```python
from build123d import *

# Parameters (mm, degrees)
F2_R         = 10
F2_R_2       = 7.5
F2_R_3       = 4.9
F3_DEPTH     = 11
F4_DEPTH     = 9
F5_DEPTH     = 18.5
F2_R_4       = 11.25
F10_DEPTH    = 1
F11_START    = 9
F10_FACE_R   = 11.25
F10_FACE_R_2 = 10
F11_DEPTH    = 1
F12_DEPTH    = 12


with BuildPart() as f3:
    # F2 (on Top) → F3 (new body)
    with BuildSketch(Plane.XY):
        Circle(F2_R)
        Circle(F2_R_2, mode=Mode.SUBTRACT)
        Circle(F2_R_2)
        Circle(F2_R_3, mode=Mode.SUBTRACT)
        Circle(F2_R_3)
        with BuildLine():
            ThreePointArc((-2.2847319318, -2.45), (-3.35, 0), (-2.2847319318, 2.45))
            Line((-2.2847319318, 2.45), (2.2847319318, 2.45))
            ThreePointArc((2.2847319318, 2.45), (3.35, 0), (2.2847319318, -2.45))
            Line((2.2847319318, -2.45), (-2.2847319318, -2.45))
        make_face(mode=Mode.SUBTRACT)
    extrude(amount=F3_DEPTH)

    # F2 (on Top) → F4 (join)
    with BuildSketch(Plane.XY):
        Circle(F2_R_2)
        Circle(F2_R_3, mode=Mode.SUBTRACT)
        Circle(F2_R_3)
        with BuildLine():
            ThreePointArc((-2.2847319318, -2.45), (-3.35, 0), (-2.2847319318, 2.45))
            Line((-2.2847319318, 2.45), (2.2847319318, 2.45))
            ThreePointArc((2.2847319318, 2.45), (3.35, 0), (2.2847319318, -2.45))
            Line((2.2847319318, -2.45), (-2.2847319318, -2.45))
        make_face(mode=Mode.SUBTRACT)
    extrude(amount=F4_DEPTH)

    # F2 (on Top) → F5 (join)
    with BuildSketch(Plane.XY):
        Circle(F2_R_3)
        with BuildLine():
            ThreePointArc((-2.2847319318, -2.45), (-3.35, 0), (-2.2847319318, 2.45))
            Line((-2.2847319318, 2.45), (2.2847319318, 2.45))
            ThreePointArc((2.2847319318, 2.45), (3.35, 0), (2.2847319318, -2.45))
            Line((2.2847319318, -2.45), (-2.2847319318, -2.45))
        make_face(mode=Mode.SUBTRACT)
    extrude(amount=F5_DEPTH)

    # F6 (on Front) → F7 (revolve)
    with BuildSketch(Plane.XZ):
        Polygon((5.15, 17.75), (4.9, 18.5), (4.9, 17), align=None)
    revolve(axis=Axis((0, 0, 8.7542282417), (0, 0, 1)))

    # F2 (on Top) → F10 (join)
    with BuildSketch(Plane.XY):
        Circle(F2_R_4)
        Circle(F2_R, mode=Mode.SUBTRACT)
    extrude(amount=F10_DEPTH)

    # F2 (on Top) + F10_face (on face) → F11 (join)
    with BuildSketch(Plane.XY.offset(F11_START)):
        Circle(F2_R)
        Circle(F2_R_2, mode=Mode.SUBTRACT)
    with BuildSketch(Plane.XY.offset(1).offset(F11_START)):
        Circle(F10_FACE_R)
        Circle(F10_FACE_R_2, mode=Mode.SUBTRACT)
    extrude(amount=F11_DEPTH)

    # F2 (on Top) → F12 (join)
    with BuildSketch(Plane.XY):
        Circle(F2_R_2)
        Circle(F2_R_3, mode=Mode.SUBTRACT)
    extrude(amount=F12_DEPTH)


solid = f3.part
```
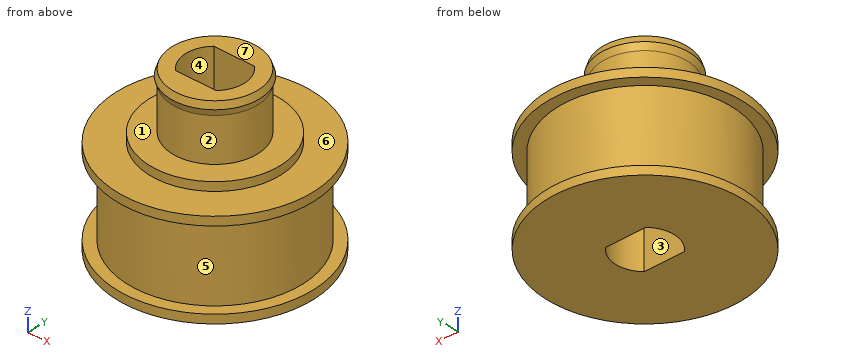
The listing builds one solid part. Answer for the finished solid, in the listing's coordinates (mm). Face numbers are marked on the shaded views. A direction names the side the tool comes from. Coordinates: 2 decimals unless noted, no trailing zeros. Loops run counter-clockwise (first coordinate to the right, second up) from the corner with the lowest first, then second, coordinate; pieces in that order, holes last. Notation, with made-up numbers: (2.25, 54.5) - (37.25, 54.5) arc R28 ccw to (37.25, 80.5) - close; hole circle Ø5 at (-27.75, 75). An arc over 180 degrees is marked (long way). Use a Markdown table: item, result. Add a question column.
1) For the marked faces 4, 5, 6 and 7, determine the directions among +Z, -Z, +X, -X, +Y, -Y from which every point of the face is accessible in a straight line to the end or side of a thin tool.
2) The part is cut by section B-B, the plane x = 0. Give the vertices of the cut face in (y, z), and give its area (3 significant figures).
3) Given pin 1 (1 mm diameter, centred on x = -8, z = 10.5, fed in from +Y); pin 2 (2.5 mm diameter, centred on x = 1, z = 6.5, fed in from -Y); pin 3 (1.5 mm diameter, centred on x = -8.5, z = 12, fed in from +Y); pin 4 (7.5 mm diameter, centred on x = 1.5, y = 1.5, fed in from +Z), each flat-ended and moving along its own axis, determine where each tip first touches the part or whether it passes through.
4) Find the intervals of material crossed by line 1 (Z direction, x = 0, y = -6); line 2 (Z direction, x = -5, y = 9.75); line 3 (Y direction, x = -0.5, z = 16.25), in increasing order.
5) The mould has two halves that part along X. Classify the marked faces 1, 2 and 3: released by +X, released by -X, zero draft, split by the parting line, or undercut.
6) The part is cut by section D-D, the plane y = -9.5. Give the vertices of the cut face in (x, z), and give its area (3 significant figures).
7) The part is cut by section C-C, the plane z = 8. Give the vertices of the cut face in (x, y).
8) The part is cut by section A-A, the plane y = 0. Give the vertices of the cut face in (x, z), and give its area (3 significant figures).
Here are the results:
| question | item | result |
|---|---|---|
| 1 | face 4 | +Z, -Z |
| 1 | face 5 | none |
| 1 | face 6 | +Z |
| 1 | face 7 | +Z, +X, -X, +Y, -Y |
| 2 | outline | (-11.25, 0) - (-2.45, 0) - (-2.45, 18.5) - (-4.9, 18.5) - (-5.15, 17.75) - (-4.9, 17) - (-4.9, 12) - (-7.5, 12) - (-7.5, 11) - (-11.25, 11) - (-11.25, 10) - (-10, 10) - (-10, 1) - (-11.25, 1) - close; (2.45, 0) - (11.25, 0) - (11.25, 1) - (10, 1) - (10, 10) - (11.25, 10) - (11.25, 11) - (7.5, 11) - (7.5, 12) - (4.9, 12) - (4.9, 17) - (5.15, 17.75) - (4.9, 18.5) - (2.45, 18.5) - close |
| 2 | area | 213 mm^2 |
| 3 | pin 1 | stops at y = 8.39 |
| 3 | pin 2 | stops at y = -10 |
| 3 | pin 3 | passes through |
| 3 | pin 4 | stops at z = 18.5 |
| 4 | line 1 | z = 0 to 12 |
| 4 | line 2 | z = 0 to 1, 10 to 11 |
| 4 | line 3 | y = -4.87 to -2.45, 2.45 to 4.87 |
| 5 | face 1 | zero draft |
| 5 | face 2 | split by the parting line |
| 5 | face 3 | undercut |
| 6 | outline | (-6.03, 0) - (6.03, 0) - (6.03, 1) - (3.12, 1) - (3.12, 10) - (6.03, 10) - (6.03, 11) - (-6.03, 11) - (-6.03, 10) - (-3.12, 10) - (-3.12, 1) - (-6.03, 1) - close |
| 6 | area | 80.3 mm^2 |
| 7 | outline | circle Ø20 at (0, 0); hole (-2.28, -2.45) - (2.28, -2.45) arc R3.35 ccw to (2.28, 2.45) - (-2.28, 2.45) arc R3.35 ccw to start |
| 8 | outline | (-11.25, 0) - (-3.35, 0) - (-3.35, 18.5) - (-4.9, 18.5) - (-5.15, 17.75) - (-4.9, 17) - (-4.9, 12) - (-7.5, 12) - (-7.5, 11) - (-11.25, 11) - (-11.25, 10) - (-10, 10) - (-10, 1) - (-11.25, 1) - close; (3.35, 0) - (11.25, 0) - (11.25, 1) - (10, 1) - (10, 10) - (11.25, 10) - (11.25, 11) - (7.5, 11) - (7.5, 12) - (4.9, 12) - (4.9, 17) - (5.15, 17.75) - (4.9, 18.5) - (3.35, 18.5) - close |
| 8 | area | 180 mm^2 |
